from build123d import *

# Parameters (mm, degrees)
SKETCH1_R           = 62.5
SKETCH1_R_2         = 37.5
BOSS_EXTRUDE1_DEPTH = 2
SKETCH2_R           = 3
CUT_EXTRUDE1_DEPTH  = 89.41097217
CIRPATTERN1_COUNT   = 3


with BuildPart() as part:
    # Sketch1 → Boss-Extrude1 (new body)
    with BuildSketch(Plane.XY):
        Circle(SKETCH1_R)
        Circle(SKETCH1_R_2, mode=Mode.SUBTRACT)
    extrude(amount=BOSS_EXTRUDE1_DEPTH)

    # Sketch2 → Cut-Extrude1 (cut, through all)
    with BuildSketch(Plane(origin=(0, 0, 0), x_dir=(-1, 0, 0), z_dir=(0, 0, -1))):
        with Locations((0, 55)):
            Circle(SKETCH2_R)
    cut_extrude1 = extrude(amount=-CUT_EXTRUDE1_DEPTH, mode=Mode.SUBTRACT)

    # CirPattern1: Cut-Extrude1 ×3 about axis
    cirpattern1_axis = Axis((0, 0, 0), (0, 0, 1))
    for i in range(1, CIRPATTERN1_COUNT):
        add(cut_extrude1.rotate(cirpattern1_axis, i * 360 / CIRPATTERN1_COUNT), mode=Mode.SUBTRACT)


solid = part.part
Could you check a few things on this model? Use its own coordinates, in mm. Give positions to 0.01 mm unless a question says otherwise; leave off trailing zeros. Order: outer loops, then holes, each group sorted by start corner. A loop starts at its lowest first (then second) coordinate and runs counter-clockwise, first axis right, second up.
Item 1: If we section it at B-B, the plane y = 0: Write out the boundary of the cut face in (x, z).
Item 2: If we section it at C-C, the plane x = -31.5: Write out the boundary of the cut face in (y, z), plus the area to 3 significant figures.
Item 3: I'm going to push flat-ended pins straight in: pin 1 (1 mm diameter, centred on y = 46.5, z = 2, fed in from -X); pin 2 (5 mm diameter, centred on x = 47.63, y = -27.5, fed in from -Z). Where does each tip first touch, or does it pass through?
Item 4: If we section it at A-A, the plane x = 0: Write out the boundary of the cut face in (y, z).
Item 5: If we mould it in two halves opening along Y, with no side actions, what happens to faces 1 (the face through (-62.44, 2.75, 0.99)), 2 (the face through (0, 58, 1)), 3 (the face through (27, -27, 2)), 4 (the face through (-4.88, 37.18, 0.99))? For each: pulls with the +Y half, pulls with the -Y half, needs draft (parallel to the pull), parting line crosses it, or undercut.
Item 6: If we section it at D-D, the plane y = -27.5: Write out the boundary of the cut face in (x, z), plus the area to 3 significant figures.
Item 7: I need wall thicknesses on line 1 (Y direction, x = 0, z = 0.8); line 2 (Y direction, x = 1, z = 1.05); line 3 (X direction, y = -28.5, z = 1.3). Which ranges of each line are inside material? Lowest first, please.
Values:
1. outline: (-62.5, 0) - (-37.5, 0) - (-37.5, 2) - (-62.5, 2) - close; (37.5, 0) - (62.5, 0) - (62.5, 2) - (37.5, 2) - close
2. outline: (-53.98, 0) - (-20.35, 0) - (-20.35, 2) - (-53.98, 2) - close; (20.35, 0) - (53.98, 0) - (53.98, 2) - (20.35, 2) - close
2. area: 135 mm2
3. pin 1: stops at x = -42.31
3. pin 2: passes through
4. outline: (-62.5, 0) - (-37.5, 0) - (-37.5, 2) - (-62.5, 2) - close; (37.5, 0) - (52, 0) - (52, 2) - (37.5, 2) - close; (58, 0) - (62.5, 0) - (62.5, 2) - (58, 2) - close
5. face 1: parting line crosses it
5. face 2: undercut
5. face 3: needs draft
5. face 4: undercut
6. outline: (-56.12, 0) - (-50.63, 0) - (-50.63, 2) - (-56.12, 2) - close; (-44.63, 0) - (-25.5, 0) - (-25.5, 2) - (-44.63, 2) - close; (25.5, 0) - (44.63, 0) - (44.63, 2) - (25.5, 2) - close; (50.63, 0) - (56.12, 0) - (56.12, 2) - (50.63, 2) - close
6. area: 98.5 mm2
7. line 1: y = -62.5 to -37.5, 37.5 to 52, 58 to 62.5
7. line 2: y = -62.49 to -37.49, 37.49 to 52.17, 57.83 to 62.49
7. line 3: x = -55.62 to -50.46, -44.8 to -24.37, 24.37 to 44.8, 50.46 to 55.62
